from build123d import *

# Parameters (mm, degrees)
F0_R     = 2.5
F0_W     = 8
F0_H     = 3.2
F0_W_2   = 3.2
F0_R_2   = 5.5
F1_DEPTH = 1.5


with BuildPart() as f1:
    # F0 (on Top) → F1 (new body, symmetric)
    with BuildSketch(Plane.XY):
        with BuildLine():
            Line((31, 22.5), (27.8, 22.5))
            Line((27.8, 22.5), (27.8, 7.5))
            Line((27.8, 7.5), (31, 7.5))
            Line((31, 7.5), (31, -7.5))
            Line((31, -7.5), (27.8, -7.5))
            Line((27.8, -7.5), (27.8, -22.5))
            Line((27.8, -22.5), (31, -22.5))
            Line((31, -22.5), (31, -32.5))
            add(Edge.make_bspline(
                [(31, -32.5), (37, -21.666667), (49, 0), (37, 21.666667), (31, 32.5)],
                knots=[0, 0, 0, 0, 34.644624, 69.289249, 69.289249, 69.289249, 69.289249], degree=3))
            Line((31, 32.5), (31, 22.5))
        make_face()
        with BuildLine():
            Line((0, 49.5), (-31, 37.5))
            add(Edge.make_bspline(
                [(-31, 37.5), (-38.6, 25), (-53.8, 0), (-38.6, -25), (-31, -37.5)],
                knots=[0, 0, 0, 0, 40.46344, 80.926881, 80.926881, 80.926881, 80.926881], degree=3))
            Line((-31, -37.5), (0, -49.5))
            Line((0, -49.5), (31, -37.5))
            add(Edge.make_bspline(
                [(31, 37.5), (38.6, 25), (53.8, 0), (38.6, -25), (31, -37.5)],
                knots=[0, 0, 0, 0, 40.46344, 80.926881, 80.926881, 80.926881, 80.926881], degree=3))
            Line((31, 37.5), (0, 49.5))
        make_face()
        with Locations((-24.5, -24)):
            Circle(F0_R, mode=Mode.SUBTRACT)
        with Locations((-17, -16.6)):
            Rectangle(F0_W, F0_H, mode=Mode.SUBTRACT)
        with Locations((-1, -16.6)):
            Rectangle(F0_W, F0_H, mode=Mode.SUBTRACT)
        with Locations((-20.4, -7.8)):
            Rectangle(F0_W_2, F0_H, mode=Mode.SUBTRACT)
        with Locations((-14, -7.8)):
            Rectangle(F0_W_2, F0_H, mode=Mode.SUBTRACT)
        with Locations((-7.6, -7.8)):
            Rectangle(F0_W_2, F0_H, mode=Mode.SUBTRACT)
        Polygon((0, -46.068615), (-22.135589, -37.5), (-21, -37.5), (-14, -37.5), (-14, -34.3), (-7, -34.3), (-7, -37.5), (0, -37.5), (0, -34.3), (7, -34.3), (7, -37.5), (14, -37.5), (14, -34.3), (21, -34.3), (21, -37.5), (22.135589, -37.5), align=None, mode=Mode.SUBTRACT)
        with Locations((24.5, -24)):
            Circle(F0_R, mode=Mode.SUBTRACT)
        with Locations((15, -16.6)):
            Rectangle(F0_W, F0_H, mode=Mode.SUBTRACT)
        with Locations((7.6, -7.8)):
            Rectangle(F0_W_2, F0_H, mode=Mode.SUBTRACT)
        with Locations((14, -7.8)):
            Rectangle(F0_W_2, F0_H, mode=Mode.SUBTRACT)
        with Locations((20.4, -7.8)):
            Rectangle(F0_W_2, F0_H, mode=Mode.SUBTRACT)
        with BuildLine():
            Line((-31, -22.5), (-31, -32.5))
            add(Edge.make_bspline(
                [(-31, 32.5), (-37, 21.666667), (-49, 0), (-37, -21.666667), (-31, -32.5)],
                knots=[0, 0, 0, 0, 34.644624, 69.289249, 69.289249, 69.289249, 69.289249], degree=3))
            Line((-31, 32.5), (-31, 22.5))
            Line((-31, 22.5), (-27.8, 22.5))
            Line((-27.8, 22.5), (-27.8, 7.5))
            Line((-27.8, 7.5), (-31, 7.5))
            Line((-31, 7.5), (-31, -7.5))
            Line((-31, -7.5), (-27.8, -7.5))
            Line((-27.8, -7.5), (-27.8, -22.5))
            Line((-27.8, -22.5), (-31, -22.5))
        make_face(mode=Mode.SUBTRACT)
        with Locations((-20.4, 7.8)):
            Rectangle(F0_W_2, F0_H, mode=Mode.SUBTRACT)
        with Locations((-14, 7.8)):
            Rectangle(F0_W_2, F0_H, mode=Mode.SUBTRACT)
        with Locations((-7.6, 7.8)):
            Rectangle(F0_W_2, F0_H, mode=Mode.SUBTRACT)
        with Locations((-17, 29.6)):
            Rectangle(F0_W, F0_H, mode=Mode.SUBTRACT)
        with Locations((-24.5, 34)):
            Circle(F0_R, mode=Mode.SUBTRACT)
        with Locations((-1, 29.6)):
            Rectangle(F0_W, F0_H, mode=Mode.SUBTRACT)
        Circle(F0_R_2, mode=Mode.SUBTRACT)
        with Locations((7.6, 7.8)):
            Rectangle(F0_W_2, F0_H, mode=Mode.SUBTRACT)
        with Locations((14, 7.8)):
            Rectangle(F0_W_2, F0_H, mode=Mode.SUBTRACT)
        with Locations((20.4, 7.8)):
            Rectangle(F0_W_2, F0_H, mode=Mode.SUBTRACT)
        with BuildLine():
            Line((27.8, 7.5), (27.8, 22.5))
            Line((27.8, 22.5), (31, 22.5))
            Line((31, 22.5), (31, 32.5))
            add(Edge.make_bspline(
                [(31, -32.5), (37, -21.666667), (49, 0), (37, 21.666667), (31, 32.5)],
                knots=[0, 0, 0, 0, 34.644624, 69.289249, 69.289249, 69.289249, 69.289249], degree=3))
            Line((31, -32.5), (31, -22.5))
            Line((31, -22.5), (27.8, -22.5))
            Line((27.8, -22.5), (27.8, -7.5))
            Line((27.8, -7.5), (31, -7.5))
            Line((31, -7.5), (31, 7.5))
            Line((31, 7.5), (27.8, 7.5))
        make_face(mode=Mode.SUBTRACT)
        with Locations((15, 29.6)):
            Rectangle(F0_W, F0_H, mode=Mode.SUBTRACT)
        with Locations((24.5, 34)):
            Circle(F0_R, mode=Mode.SUBTRACT)
        Polygon((22.135589, 37.5), (0, 37.5), (-22.135589, 37.5), (0, 46.068615), align=None, mode=Mode.SUBTRACT)
    extrude(amount=F1_DEPTH, both=True)


solid = f1.part
Read the model definition and answer for the solid it produces. Units are mm, in the model's axes. Coordinates: 2 decimals unless noted, no trailing zeros. Order: outer loops, then holes, each group sorted by start corner. A loop starts at its lowest first (then second) coordinate and runs counter-clockwise, first axis right, second up. Notation, with made-up numbers: (-24.75, 62) - (-10.75, 62) arc R24 cw to (-10.75, 75) - close; hole circle Ø10 at (14, 82.5). An arc over 180 degrees is marked (long way). Use one line per item in the form item = value.
(1) For a pull along X with two mould halves and no side action, classify faces 1 (the face through (9.2, -8, 0)), 2 (the face through (-1, -10, -1.5)), 3 (the face through (15.283, -43.584, 0.021)) as pulls with the +X half, pulls with the -X half, needs draft (parallel to the pull), parting line crosses it, or undercut.
Computed values:
face_1 = undercut
face_2 = needs draft
face_3 = pulls with the +X half
(2) Straight lines are drawn through the part: L1, parallel to X at y = 26.5, z = -1.2; L2, parallel to X at y = -14, z = -0.95; L3, parallel to Y at x = -24.5, z = -0.55. For each, find the intervals that lie inside material, in ascending order.
Computed values:
L1 = -37.5 to -34.29, -31 to 31, 34.29 to 37.5
L2 = -43.42 to -40.14, -27.8 to 27.8, 40.14 to 43.42
L3 = -40.02 to -26.5, -21.5 to 31.5, 36.5 to 40.02
(3) Section A-A, the plane x = -11 is taken. Give the vertices of the cut face in (y, z), then the cut area to 3 significant figures.
Computed values:
outline = (-45.24, -1.5) - (-41.81, -1.5) - (-41.81, 1.5) - (-45.24, 1.5) - close; (-34.3, -1.5) - (37.5, -1.5) - (37.5, 1.5) - (-34.3, 1.5) - close; (41.81, -1.5) - (45.24, -1.5) - (45.24, 1.5) - (41.81, 1.5) - close
area = 236 mm²
(4) Section B-B, the plane y = -35.5 is taken. Give the number of separate pieces and of enclosed holes in the cut face, then the cut area to 3 significant figures.
Computed values:
separate_pieces = 4
enclosed_holes = 0
area = 130 mm²
(5) Given pin 1 Ø1.5 at (y, z) = (-36.5, 0) entering from -X; pin 2 Ø1 at (y, z) = (-12, 0.5) entering from +X (3 decimals); pin 3 Ø1.5 at (x, z) = (14, 0.5) entering from -Y, each flat-ended and moving along its own axis, determine where each tip first touches the part or whether it passes through.
Computed values:
pin_1 = -32.06
pin_2 = 44.275
pin_3 = -44.37
